The listing builds one solid part. Answer for the finished solid, in the listing's coordinates (mm). A direction names the side the tool comes from. Give positions to 0.01 mm unless a question says otherwise; leave off trailing zeros. Loops run counter-clockwise (first coordinate to the right, second up) from the corner with the lowest first, then second, coordinate; pieces in that order, holes last.
Item 1: The mould has two halves that part along Z. Classify faces 1 (the face through (-37.257, 19.72, 28.665)), 2 (the face through (40.146, 19.72, -24.404)), 3 (the face through (-11.49, 20.28, 34.34)): pulls with the +Z half, pulls with the -Z half, needs draft (parallel to the pull), parting line crosses it, or undercut.
Item 2: Section A-A, the plane x = -27 is taken. Give the vertices of the cut face in (y, z), and give its area (3 significant figures).
Item 3: Consider line 1 along X through (y, z) = (24, -41.5); line 2 along X through (y, z) = (30, -40.5); line 3 along X through (y, z) = (5, 43). Determine where each line is inside the solid, lowest interval first.
Item 4: Each of these flat-tipped pins is pushed along its axis until it touches: pin 1 Ø12 at (y, z) = (19.5, -18.5) entering from +X; pin 2 Ø12 at (x, y) = (-20, 12.5) entering from -Z; pin 3 Ø1 at (y, z) = (25, 15.5) entering from +X. Where does it stop, or does it pass through?
Item 5: A tool of negligible diameter and unlimited length cuts with its end or side. For faces 4 (the face through (36.174, 20.28, 1.649)), 5 (the face through (-23.12, 20.28, 27.87)), 6 (the face through (-26.166, 20.28, -31.555)), from which of +Z, -Z, +X, -X, +Y, -Y can it reach the whole face along a straight path? Write none if from no direction.
from build123d import *

# Parameters (mm, degrees)
ENL_V_MAT_EXTRU_3_DEPTH            = 79.182478856
CONG_1_R                           = 2.5
R_P_TITION_CIRCULAIRE1_COUNT       = 17
CONG_1_OF_R_P_TITION_CIRCULAIRE1_R = 2.5
ENL_V_MAT_EXTRU_4_DEPTH            = 79.135714235


with BuildPart() as part:
    # Esquisse1 → Révolution1 (revolve)
    with BuildSketch(Plane.XY, mode=Mode.PRIVATE) as r_volution1_sk:
        Polygon((-47.5, 40), (-47.5, 0), (-40, 0), (0, 0), (0, 40), (-40, 40), align=None)
    revolve(r_volution1_sk.sketch.rotate(Axis((0, 40, 0), (0, -1, 0)), 270), axis=Axis((0, 40, 0), (0, -1, 0)))

    # Esquisse5 → Enlèv. mat.-Extru.3 (cut, through all)
    with BuildSketch(Plane(origin=(0, 40, 0), x_dir=(1, 0, 0), z_dir=(0, 1, 0))):
        with BuildLine():
            ThreePointArc((-4.382747075, 47.297373374), (-10.875151123, 46.238307582), (-17.158979144, 44.292430897))
            Line((-17.158979144, 44.292430897), (-9.920283391, 34.866179565))
            Line((-9.920283391, 34.866179565), (-6.660920021, 35.632774863))
            Line((-6.660920021, 35.632774863), (-4.382747075, 47.297373374))
        make_face()
    enl_v_mat_extru_3 = extrude(amount=-ENL_V_MAT_EXTRU_3_DEPTH, mode=Mode.SUBTRACT)

    # Congé1
    cong_1_edges = [part.edges().sort_by_distance(p)[0] for p in [
        (-17.158979144, 20, -44.292430897),
        (-4.382747075, 20, -47.297373374),
    ]]
    fillet(cong_1_edges, radius=CONG_1_R)

    # Répétition circulaire1: Enlèv. mat.-Extru.3 ×17 about axis
    r_p_tition_circulaire1_axis = Axis((0, 0, 0), (0, 1, 0))
    for i in range(1, R_P_TITION_CIRCULAIRE1_COUNT):
        add(enl_v_mat_extru_3.rotate(r_p_tition_circulaire1_axis, i * 360 / R_P_TITION_CIRCULAIRE1_COUNT), mode=Mode.SUBTRACT)

    # Congé1 of Répétition circulaire1
    cong_1_of_r_p_tition_circulaire1_edges = [part.edges().sort_by_distance(p)[0] for p in [
        (-32.000543073, 20, -35.102923568),
        (-21.1725719, 20, -42.520256339),
        (-42.520256339, 20, -21.172571899),
        (-35.102923568, 20, -32.000543073),
        (-47.297373374, 20, -4.382747075),
        (-44.292430897, 20, -17.158979144),
        (-45.686718051, 20, 12.998992028),
        (-47.5, 20, 0),
        (-37.905818296, 20, 28.625145228),
        (-44.292430897, 20, 17.158979144),
        (-25.005527737, 20, 40.385313947),
        (-35.102923568, 20, 32.000543073),
        (-8.728102096, 20, 46.691222235),
        (-21.172571899, 20, 42.52025634),
        (8.728102096, 20, 46.691222235),
        (-4.382747074, 20, 47.297373374),
        (25.005527737, 20, 40.385313947),
        (12.998992029, 20, 45.686718051),
        (37.905818296, 20, 28.625145228),
        (28.625145228, 20, 37.905818296),
        (45.686718051, 20, 12.998992028),
        (40.385313947, 20, 25.005527736),
        (47.297373374, 20, -4.382747075),
        (46.691222235, 20, 8.728102096),
        (42.520256339, 20, -21.172571899),
        (46.691222235, 20, -8.728102097),
        (32.000543073, 20, -35.102923568),
        (40.385313947, 20, -25.005527737),
        (17.158979144, 20, -44.292430897),
        (28.625145228, 20, -37.905818296),
        (0, 20, -47.5),
        (12.998992028, 20, -45.686718051),
    ]]
    fillet(cong_1_of_r_p_tition_circulaire1_edges, radius=CONG_1_OF_R_P_TITION_CIRCULAIRE1_R)

    # Esquisse6 → Enlèv. mat.-Extru.4 (cut, through all)
    with BuildSketch(Plane(origin=(0, 40, 0), x_dir=(1, 0, 0), z_dir=(0, 1, 0))):
        with BuildLine():
            Line((-12.296722124, 3.175), (-15.496722124, 3.175))
            Line((-15.496722124, 3.175), (-15.496722124, -3.175))
            Line((-15.496722124, -3.175), (-12.296722124, -3.175))
            ThreePointArc((-12.296722124, -3.175), (12.7, 0), (-12.296722124, 3.175))
        make_face()
    extrude(amount=-ENL_V_MAT_EXTRU_4_DEPTH, mode=Mode.SUBTRACT)


solid = part.part
Worked answers:
1. face 1: undercut
1. face 2: pulls with the -Z half
1. face 3: pulls with the +Z half
2. outline: (0, -32.06) - (40, -32.06) - (40, 28.05) - (0, 28.05) - close
2. area: 2,400 mm2
3. line 1: x = -20.84 to -15.01, -5.52 to 1.76, 10.36 to 16.92
3. line 2: x = -20.81 to -14.25, -5.71 to 2.05, 9.73 to 16.84
3. line 3: x = -9.1 to -2.68, 6.85 to 13.02
4. pin 1: stops at x = 41.92
4. pin 2: stops at z = -43.75
4. pin 3: stops at x = 32.96
5. face 4: +X, +Y, -Y
5. face 5: +Y, -Y
5. face 6: -Z, +Y, -Y
